```python
from build123d import *

# Parameters (mm, degrees)
SKETCH_1_W      = 15
SKETCH_1_H      = 100
EXTRUDE_1_DEPTH = 80
FILLET_1_R      = 3
FILLET_2_R      = 3


with BuildPart() as part:
    # 스케치1 → 보스-돌출1 (new body)
    with BuildSketch(Plane(origin=(0, 0, 0), x_dir=(0, 0, -1), z_dir=(1, 0, 0))):
        Polygon((0, -10), (0, 0), (100, 0), (100, 100), (110, 100), (110, -10), align=None)
        with Locations((102.5, -60)):
            Rectangle(SKETCH_1_W, SKETCH_1_H)
        with Locations((7.5, -60)):
            Rectangle(SKETCH_1_W, SKETCH_1_H)
    extrude(amount=EXTRUDE_1_DEPTH)

    # 필렛1
    fillet_1_edges = [part.edges().sort_by_distance(p)[0] for p in [
        (0, 100, -105),
        (80, 100, -105),
    ]]
    fillet(fillet_1_edges, radius=FILLET_1_R)

    # 필렛2
    fillet_2_edges = [part.edges().sort_by_distance(p)[0] for p in [
        (0, -55, 0),
        (80, -55, 0),
    ]]
    fillet(fillet_2_edges, radius=FILLET_2_R)


solid = part.part
```
Input: part model. Units: mm. Frame: model coordinates. A direction names the side the tool comes from. Round coordinates to 2 decimals unless told otherwise and drop trailing zeros. Loops run counter-clockwise (first coordinate to the right, second up) from the corner with the lowest first, then second, coordinate; pieces in that order, holes last.
1) Section query A-A on y = -68.5. Return the cut outline in (x, z).
Ans:
outline: (0, -110) - (80, -110) - (80, -95) - (0, -95) - close; (0, -15) - (80, -15) - (80, -3) arc R3 ccw to (77, 0) - (3, 0) arc R3 ccw to (0, -3) - close
2) Section query B-B on x = 32. Return the cut outline in (y, z).
Ans:
outline: (-110, -110) - (100, -110) - (100, -100) - (0, -100) - (0, 0) - (-110, 0) - (-110, -15) - (-10, -15) - (-10, -95) - (-110, -95) - close
3) Material intervals for line 1 (Z direction, x = 29.5, y = -16); line 2 (Z direction, x = 56, y = 2.5); line 3 (Y direction, x = 25, z = -4.5), sorted ascending.
Ans:
line 1: z = -110 to -95, -15 to 0
line 2: z = -110 to -100
line 3: y = -110 to 0
4) Set-up query: faces 4 (the flat face through (39, -61, -15)), 5 (the flat face through (39, 0, -49)), 6 (the flat face through (80, -6, -69)). Return all of +Z, -Z, +X, -X, +Y, -Y with unobstructed straight access to the full face (end or side cutting, diameter ignored); none if empty.
Ans:
face 4: +X, -X, -Y
face 5: +Z, +X, -X, +Y
face 6: +Z, -Z, +X, +Y, -Y
5) Section query C-C on z = -10.5. Return the cut outline in (x, y), plus the area to 3 significant figures.
Ans:
outline: (0, -110) - (80, -110) - (80, 0) - (0, 0) - close
area: 8,800 mm2
6) Section query D-D on y = 38. Return the cut outline in (x, z), plus the area to 3 significant figures.
Ans:
outline: (0, -110) - (80, -110) - (80, -100) - (0, -100) - close
area: 800 mm2
7) Pin query (flat end, axial travel): pin 1 (24 mm diameter, centred on x = 22.5, z = -35.5, fed in from +Y); pin 2 (3 mm diameter, centred on x = 40.5, y = 39, fed in from +Z); pin 3 (3 mm diameter, centred on y = -69.5, z = -97, fed in from -X). Return the tip coordinate at first contact, or that it passes through.
Ans:
pin 1: stops at y = 0
pin 2: stops at z = -100
pin 3: stops at x = 0
8) Pull-direction query (Z, two-part tool) for faces 1 (the flat face through (39, -54, 0)), 2 (the flat face through (39, -61, -95)), 3 (the flat face through (39, 100, -105)); classes: released by +Z, released by -Z, zero draft, split by the parting line, or undercut.
Ans:
face 1: released by +Z
face 2: undercut
face 3: zero draft
